from build123d import *

# Parameters (mm, degrees)
SKETCH6_W                     = 2.25
SKETCH6_H                     = 12
M4_CLEARANCE_HOLE1_AT_2_COUNT = 2
M4_CLEARANCE_HOLE1_AT_2_PITCH = 148.408220797
CUT_EXTRUDE1_START            = -24
CUT_EXTRUDE1_DEPTH            = 26


with BuildPart() as part:
    # Sweep1: sweep along a path in Sketch1
    with BuildLine(Plane(origin=(0, 152.68757152, 0), x_dir=(1, 0, 0), z_dir=(0, 1, 0))) as sweep1_path:
        Line((82.38365074, -11.079514347), (82.38365074, -76.079514347))
        ThreePointArc((82.38365074, -76.079514347), (70.301805464, -105.247669071), (41.13365074, -117.329514347))
        Line((41.13365074, -117.329514347), (-46.36634926, -117.329514347))
        ThreePointArc((-46.36634926, -117.329514347), (-75.534503984, -105.247669071), (-87.61634926, -76.079514347))
        Line((-87.61634926, -76.079514347), (-87.61634926, 1.420485653))
        ThreePointArc((-87.61634926, 1.420485653), (-75.534503984, 30.588640377), (-46.36634926, 42.670485653))
        Line((-46.36634926, 42.670485653), (-16.36634926, 42.670485653))
    # Sketch2 → Sweep1 (sweep)
    with BuildSketch(Plane.ZY.offset(52.61634926)):
        Polygon((-45.670485653, 153.211679549), (-45.670485653, 158.68757152), (-39.670485653, 158.68757152), (-39.670485653, 148.68757152), (-39.670485653, 142.68757152), (-39.670485653, 122.68757152), (-45.670485653, 122.68757152), (-45.670485653, 142.68757152), align=None)
    sweep(path=sweep1_path.line)

    # Sketch6 → M4 Clearance Hole1 (revolve, cut)
    with BuildSketch(Plane(origin=(-42.61634926, 146.68757152, -42.670485653), x_dir=(0, 0, -1), z_dir=(1, 0, 0))):
        with Locations((1.125, 6)):
            Rectangle(SKETCH6_W, SKETCH6_H)
    m4_clearance_hole1 = revolve(axis=Axis((-42.61634926, 140.33757152, -42.670485653), (0, 1, 0)), mode=Mode.SUBTRACT)

    # M4 Clearance Hole1 at 2: M4 Clearance Hole1 ×2
    with Locations(*[Vector(0.8422714006615114, 0, 0.5390536964233672) * (i * M4_CLEARANCE_HOLE1_AT_2_PITCH) for i in range(1, M4_CLEARANCE_HOLE1_AT_2_COUNT)]):
        add(m4_clearance_hole1, mode=Mode.SUBTRACT)

    # Sketch7 → Cut-Extrude1 (cut)
    with BuildSketch(Plane(origin=(0, 148.68757152, 0), x_dir=(1, 0, 0), z_dir=(0, 1, 0)).offset(CUT_EXTRUDE1_START)):
        Polygon((79.889021707, -75.697125548), (85.819751318, -76.606216457), (85.819751318, -11.606216457), (79.889021707, -10.697125548), align=None)
        with BuildLine():
            Line((-46.748738059, 40.17585662), (-16.748738059, 40.17585662))
            Line((-16.748738059, 40.17585662), (-15.83964715, 46.106586231))
            Line((-15.83964715, 46.106586231), (-45.83964715, 46.106586231))
            ThreePointArc((-45.83964715, 46.106586231), (-52.06795996, 45.744481811), (-58.185151135, 44.518524149))
            Line((-58.185151135, 44.518524149), (-56.61634926, 38.797784913))
            ThreePointArc((-56.61634926, 38.797784913), (-51.727010908, 39.805226198), (-46.748738059, 40.17585662))
        make_face()
    extrude(amount=CUT_EXTRUDE1_DEPTH, mode=Mode.SUBTRACT)


solid = part.part
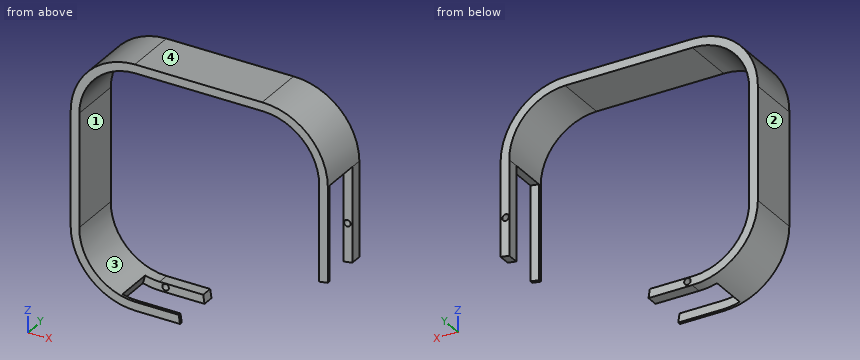
CAD build for the part. Positions are in the model's coordinates, mm. Face numbers are marked on the shaded views. Give positions to 0.01 mm unless a question says otherwise; leave off trailing zeros. Loops run counter-clockwise (first coordinate to the right, second up) from the corner with the lowest first, then second, coordinate; pieces in that order, holes last. Notation, with made-up numbers: M 73,-28 L 103,-28 A31 ccw 103,-2 Z; hole C 64,28.5 d10. An arc over 180 degrees is marked long. Answer in a Markdown table with one row per item. Add a question column.
Item 1: Drop flat-ended pins along their axis: P1, Ø9, axis at y = 156, z = 56.5, coming from the -X side; P2, Ø1.6, axis at x = -28, y = 123.5, coming from the -Z side; P3, Ø3, axis at x = 65, y = 128.5, coming from the -Z side. Give the stop position or say it passes through.
Item 2: Band-saw the part on D-D on y = 146. Give the cut face in (x, z).
Item 3: Mould opens along X. For the marked faces 1, 2, 3 and 4 say: +X half, -X half, draft (parallel to the pull), parting line (faces both ways), or undercut.
Item 4: Probe probe 1 along Z at (x, y) = (-19, 151.5); probe 2 along X at (y, z) = (129.5, 11); probe 3 along Z at (x, y) = (-12, 126.5). List the from-to ranges inside material, lowest first.
Item 5: Band-saw the part on C-C on z = 88. Give the cut face in (x, y).
Item 6: Band-saw the part on B-B on z = 31.5. Give the cut face in (x, y).
Item 7: Band-saw the part on A-A on x = -38. Give the cut face in (y, z).
Reply:
| question | item | result |
|---|---|---|
| 1 | P1 | stops at x = -91.05 |
| 1 | P2 | stops at z = -46.11 |
| 1 | P3 | stops at z = 105.38 |
| 2 | outline | M -91.05,-1.95 A44.69 ccw -58.19,-44.52 L -56.62,-38.8 A38.76 cw -85.12,-1.04 L -85.12,76.46 A38.76 cw -45.98,114.83 L 41.52,114.83 A38.76 cw 79.89,75.7 L 85.82,76.61 A44.69 ccw 40.61,120.77 L -46.89,120.77 A44.69 ccw -91.05,75.55 Z |
| 3 | face 1 | undercut |
| 3 | face 2 | -X half |
| 3 | face 3 | +X half |
| 3 | face 4 | draft |
| 4 | probe 1 | z = -46.11 to -40.18, 114.83 to 120.77 |
| 4 | probe 2 | x = -91.05 to -85.12 |
| 4 | probe 3 | z = 114.83 to 120.77 |
| 5 | outline | M -89.44,122.69 L -83.24,122.69 L -83.24,158.69 L -89.44,158.69 Z; M 78.01,122.69 L 84.2,122.69 L 84.2,158.69 L 78.01,158.69 Z |
| 6 | outline | M -91.05,122.69 L -85.12,122.69 L -85.12,158.69 L -91.05,158.69 Z; M 79.89,122.69 L 85.82,122.69 L 85.82,124.69 L 79.89,124.69 Z; M 79.89,150.69 L 85.82,150.69 L 85.82,158.69 L 79.89,158.69 Z |
| 7 | outline | M 122.69,-46.11 L 124.69,-46.11 L 124.69,-40.18 L 122.69,-40.18 Z; M 122.69,114.83 L 158.69,114.83 L 158.69,120.77 L 122.69,120.77 Z; M 150.69,-46.11 L 158.69,-46.11 L 158.69,-40.18 L 150.69,-40.18 Z |
